Here's the drawing with two shaded views (mm, measured from the low corner). I have some questions. A direction names the side the tool comes from. Round coordinates to 2 decimals unless told otherwise and drop trailing zeros. Loops run counter-clockwise (first coordinate to the right, second up) from the corner with the lowest first, then second, coordinate; pieces in that order, holes last. Notation, with made-up numbers: (14, 20.5) -> (32, 20.5) arc R17 cw to (32, 52.5) -> close; hole circle Ø10 at (2.5, 47.25). An arc over 180 degrees is marked (long way). Write each question's results on one line, items separated by ' | '. Start each with the question number.
1) Imagine slicing it at A-A, the plane z = 15. List the corners of the cut face in (x, y) for me.
2) Imagine slicing it at D-D, the plane z = 3. List the corners of the cut face in (x, y) for me.
3) For P1, Ø12, axis at y = 33, z = 4.5, coming from the -X side; P2, Ø2, axis at y = 48, z = 6, coming from the +X side, each with a flat end and sliding along its axis, tell me the tip position at first contact or that it passes through.
4) Imagine slicing it at C-C, the plane x = 53.5. List the corners of the cut face in (y, z) for me, plus the area to 3 significant figures.
5) Which directions (+Z, -Z, +X, -X, +Y, -Y) give clear straight access to the entire face, cutting with the end or side of a thin tool? Please do the marked faces 1 and 2.
6) If I drill on probe 1 along X at (y, z) = (60.5, 16); probe 2 along Z at (x, y) = (56.5, 35); probe 3 along X at (y, z) = (14.5, 9), over which ranges is the centre line in solid material (lowest first)?
7) Imagine slicing it at B-B, the plane y = 42. List the corners of the cut face in (x, z) for me.
8) We'd pull the mould along X, two halves only. Please class the marked faces 3, 4, 5 and 6: pulls with the +X half, pulls with the -X half, needs draft (parallel to the pull), parting line crosses it, or undercut.
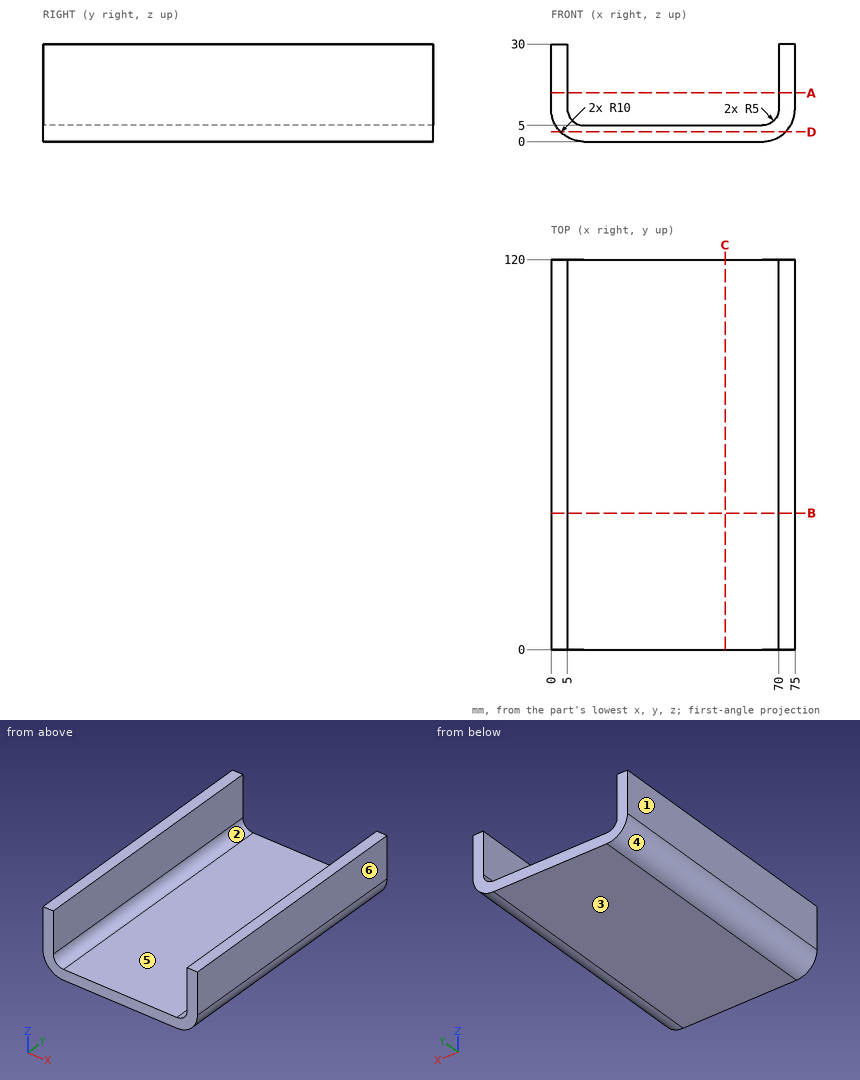
Checked values:
1) outline: (0, 0) -> (5, 0) -> (5, 120) -> (0, 120) -> close; (70, 0) -> (75, 0) -> (75, 120) -> (70, 120) -> close
2) outline: (2.86, 0) -> (72.14, 0) -> (72.14, 120) -> (2.86, 120) -> close
3) P1: x = 0 | P2: x = 74.54
4) outline: (0, 0) -> (120, 0) -> (120, 5) -> (0, 5) -> close | area: 600 mm^2
5) face 1: +Z, -Z, -X, +Y, -Y | face 2: +Z, +Y, -Y
6) probe 1: 0 to 5, 70 to 75 | probe 2: 0 to 5 | probe 3: 0.05 to 5.1, 69.9 to 74.95
7) outline: (0, 10) arc R10 ccw to (10, 0) -> (65, 0) arc R10 ccw to (75, 10) -> (75, 30) -> (70, 30) -> (70, 10) arc R5 cw to (65, 5) -> (10, 5) arc R5 cw to (5, 10) -> (5, 30) -> (0, 30) -> close
8) face 3: needs draft | face 4: pulls with the -X half | face 5: undercut | face 6: pulls with the +X half
